Design review of the part built by this model. Coordinates are the model's own, in mm. A direction names the side the tool comes from. Coordinates: 2 decimals unless noted, no trailing zeros. Loops run counter-clockwise (first coordinate to the right, second up) from the corner with the lowest first, then second, coordinate; pieces in that order, holes last. Notation, with made-up numbers: M 74.25,61 L 115.25,61 A20 ccw 115.25,83 Z; hole C 31,30 d3. An arc over 180 degrees is marked long. Write item = value, one per line. Start each with the question number.
from build123d import *

# Parameters (mm, degrees)
F2_DEPTH = 1000
F3_W     = 940
F3_H     = 277.328980073
F4_DEPTH = 5
F6_D     = 145
F6_DEPTH = 4
F6_TIP   = 43.5623948795
F1_W     = 200
F1_H     = 70
F7_DEPTH = 2
F8_W     = 201.8966459586
F8_H     = 70
F9_DEPTH = 2


with BuildPart() as f2:
    # F1 (on Right) → F2 (new body)
    with BuildSketch(Plane.YZ):
        Polygon((-288.5542339748, 27.2076225815), (-288.5542339748, -222.7923774185), (311.4457660252, -222.7923774185), (311.4457660252, 247.2076225815), (-8.5542339748, 249.2076225815), align=None)
        Polygon((-286.5542339748, 26.2409870095), (-7.8630740966, 247.2032637701), (309.4457660252, 245.2200835194), (309.4457660252, -220.7923774185), (-286.5542339748, -220.7923774185), align=None, mode=Mode.SUBTRACT)
    extrude(amount=F2_DEPTH)

    # F3 (on face) → F4 (cut)
    with BuildSketch(Plane(origin=(0, -124.6227615588, 157.1818614256), x_dir=(1, 0, 0), z_dir=(0, -0.6212762255, 0.7835916358))):
        with Locations((500, -40.5407451073)):
            Rectangle(F3_W, F3_H)
    extrude(amount=-F4_DEPTH, mode=Mode.SUBTRACT)

    # F6
    with Locations(Plane.XZ.offset(288.5542339748)):
        with Locations((120, -62.7923774185), (500, -62.7923774185), (880, -62.7923774185)):
            Hole(F6_D / 2, depth=F6_DEPTH)
            with Locations((0, 0, -(F6_DEPTH + F6_TIP / 2))):  # 118° drill point
                Cone(0, F6_D / 2, F6_TIP, mode=Mode.SUBTRACT)

    # F1 (on Right) → F7 (join)
    with BuildSketch(Plane.YZ):
        Polygon((309.4457660252, 245.2200835194), (-7.8630740966, 247.2032637701), (-286.5542339748, 26.2409870095), (-286.5542339748, -220.7923774185), (309.4457660252, -220.7923774185), align=None)
        with Locations((-86.5542339748, -67.7923774185)):
            Rectangle(F1_W, F1_H, mode=Mode.SUBTRACT)
    extrude(amount=F7_DEPTH)

    # F8 (on face) → F9 (join)
    with BuildSketch(Plane.YZ.offset(1000)):
        Polygon((-288.4508799334, 27.2547214809), (-288.4508799334, -222.7452785191), (311.5491200666, -222.7452785191), (311.5491200666, 247.2547214809), (-8.4508799334, 247.2547214809), align=None)
        with Locations((-87.5025569541, -67.7452785191)):
            Rectangle(F8_W, F8_H, mode=Mode.SUBTRACT)
    extrude(amount=F9_DEPTH)


solid = f2.part
Q1. Mouldability with a two-part tool opening along Z and no side actions: class faces 4 (the face through (30, -157, 130)), 5 (the face through (493, 7, -222.792)), 6 (the face through (50.848, -287.54, -41.015)) as released by +Z, released by -Z, zero draft, split by the parting line, or undercut.
Q2. Add section D-D on x = 307. State the section outline as (y, z) points, plus the area to 3 significant figures.
Q3. To check wall thickness, follow line 1 (Y direction, x = 646, z = -196.5); line 2 (X direction, y = -98.5, z = 41); line 3 (Z direction, x = 126, y = -132). State the ranges of each line that lie inside material, in increasing order. Write a range as from..to.
Q4. Clearance check with flat-ended pins moving along their axes: P1, Ø1, axis at x = 428.5, z = -80.5, coming from the +Y side; P2, Ø1.6, axis at x = 1001, z = -35, coming from the -Y side; P3, Ø0.6, axis at x = 0.5, y = -127.5, coming from the +Z side. State where each tip first meets the part, or that it passes through.
Q5. For faces 1 (the face through (2, 73, 16)), 2 (the face through (1000.986, -146.491, 138.795)), 3 (the face through (810.848, -287.54, -41.015)), list the 3-axis set-ups (+Z, -Z, +X, -X, +Y, -Y) from which the entire face can be reached by the end or side of a thin tool; tool diameter is ignored.
Q6. Add section B-B on y = 26.5. State the section outline as (x, z) points.
Q7. Add section A-A on x = 500. State the section outline as (y, z) points.
Q8. Add section C-C on z = 136.5. State the section outline as (x, y) points.
Values follow:
q1.face_4 = zero draft
q1.face_5 = released by -Z
q1.face_6 = undercut
q2.outline = M -288.55,-222.79 L 311.45,-222.79 L 311.45,247.21 L -8.55,249.21 L -47.73,218.14 L -46.49,216.58 L -7.86,247.2 L 309.45,245.22 L 309.45,-220.79 L -286.55,-220.79 L -286.55,26.24 L -263.8,44.28 L -265.05,45.85 L -288.55,27.21 Z
q2.area = 3,420 mm2
q3.line_1 = -288.55..-286.55, 309.45..311.45
q3.line_2 = 0..2, 1000..1002
q3.line_3 = -222.79..-220.79
q4.P1 = 311.45
q4.P2 = -288.45
q4.P3 = 155.14
q5.face_1 = none
q5.face_2 = +Z, +X, -Y
q5.face_3 = -Y
q6.outline = M 0,-222.79 L 1000,-222.79 L 1000,-222.75 L 1002,-222.75 L 1002,247.25 L 1000,247.25 L 1000,248.99 L 0,248.99 Z; hole M 2,-220.79 L 1000,-220.79 L 1000,246.99 L 2,246.99 Z
q7.outline = M -288.55,-222.79 L 311.45,-222.79 L 311.45,247.21 L -8.55,249.21 L -47.73,218.14 L -46.49,216.58 L -7.86,247.2 L 309.45,245.22 L 309.45,-220.79 L -286.55,-220.79 L -286.55,-135.29 L -288.55,-135.29 Z; M -288.55,9.71 L -286.55,9.71 L -286.55,26.24 L -263.8,44.28 L -265.05,45.85 L -288.55,27.21 Z
q8.outline = M 0,-150.71 L 30,-150.71 L 30,-147.49 L 2,-147.49 L 2,309.45 L 1000,309.45 L 1000,-147.49 L 970,-147.49 L 970,-150.71 L 1000,-150.71 L 1000,-149.41 L 1002,-149.41 L 1002,311.55 L 1000,311.55 L 1000,311.45 L 0,311.45 Z
